The listing builds one solid part. Answer for the finished solid, in the listing's coordinates (mm). Face numbers are marked on the shaded views. A direction names the side the tool comes from. Round coordinates to 2 decimals unless told otherwise and drop trailing zeros. Order: outer loops, then holes, each group sorted by start corner. A loop starts at its lowest first (then second) coordinate and runs counter-clockwise, first axis right, second up. Notation, with made-up numbers: (39.5, -7) - (66.5, -7) arc R25 ccw to (66.5, 13) - close; hole circle Ø2 at (39.5, -17). An arc over 180 degrees is marked (long way). One line per item, written item: value. Start each with the question number.
1. A tool of negligible diameter and unlimited length cuts with its end or side. For the marked faces 1, 2 and 3, from which of +Z, -Z, +X, -X, +Y, -Y can it reach the whole face along a straight path? Write none if from no direction.
2. Straight lines are drawn through the part: line 1 (X direction, y = 1, z = 1.75); line 2 (Y direction, x = 21, z = 2.5); line 3 (Z direction, x = 51.5, y = 2). For each, find the intervals that lie inside material, in ascending order.
3. Section C-C, the plane x = -70 is taken. Give the vertices of the cut face in (y, z), then the cut area to 3 significant figures.
4. Flat-ended cylindrical pins translate along their axes: P1, Ø9, axis at x = 56.77, y = -1.58, coming from the -Z side; P2, Ø0.8, axis at y = 7, z = 3, coming from the +X side; P3, Ø1.5, axis at x = -102.5, z = 4.5, coming from the +Y side; P4, Ø1.2, axis at y = 7, z = 6, coming from the -X side. Find the tip coordinate at first contact, or state that the pin passes through.
5. Section B-B, the plane x = 42 is taken. Give the vertices of the cut face in (y, z).
6. Section A-A, the plane z = 3.25 is taken. Give the vertices of the cut face in (x, y) (3 decimals).
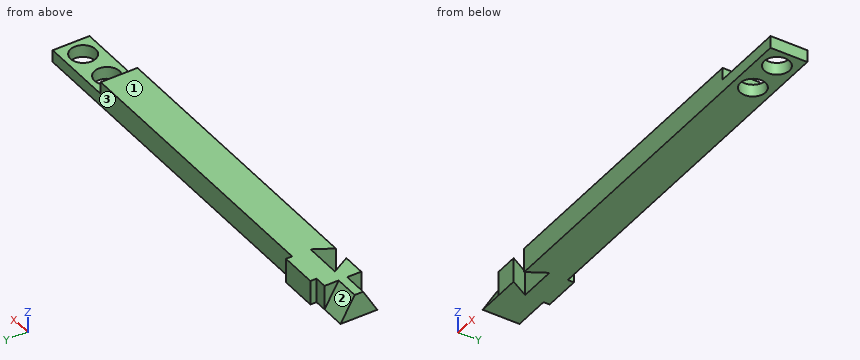
from build123d import *

# Parameters (mm, degrees)
SKETCH_W        = 170
SKETCH_H        = 15
PAD_DEPTH       = 10
SKETCH001_W     = 35
SKETCH001_H     = 25
POCKET_DEPTH    = 5
PAD002_DEPTH    = 10
POCKET001_DEPTH = 10
SKETCH002_R     = 5.125
POCKET002_DEPTH = 5
SKETCH005_W     = 15.25
SKETCH005_H     = 10
PAD003_DEPTH    = 2.5


with BuildPart() as part:
    # Sketch → Pad (new body)
    with BuildSketch(Plane.XY):
        with Locations((-20.728933, -1.58076)):
            Rectangle(SKETCH_W, SKETCH_H)
    extrude(amount=PAD_DEPTH)

    # Sketch001 (on Face6 of Pad) → Pocket (cut)
    with BuildSketch(Plane.XY.offset(10)):
        with Locations((51.771067, -1.58076)):
            Rectangle(SKETCH001_W, SKETCH001_H)
    extrude(amount=-POCKET_DEPTH, mode=Mode.SUBTRACT)

    # Sketch003 → Pad002 (join)
    with BuildSketch(Plane(origin=(-105.728933, 0, 0), x_dir=(0, -1, 0), z_dir=(-1, 0, 0))):
        Polygon((-5.91924, 0), (-0.145737, 10), (3.307257, 10), (9.08076, 0), align=None)
    extrude(amount=PAD002_DEPTH)

    # Sketch004 (on Face3 of Pad002) → Pocket001 (cut)
    with BuildSketch(Plane.XY.offset(10)):
        Polygon((-93.103933, -14.787648), (-100.728933, -1.58076), (-85.478933, -1.58076), align=None)
    extrude(amount=-POCKET001_DEPTH, mode=Mode.SUBTRACT)

    # Sketch002 (on Face7 of Pocket) → Pocket002 (cut)
    with BuildSketch(Plane.XY.offset(5)):
        with Locations((56.771067, -1.58076)):
            Circle(SKETCH002_R)
        with Locations((41.771067, -1.58076)):
            Circle(SKETCH002_R)
    extrude(amount=-POCKET002_DEPTH, mode=Mode.SUBTRACT)

    # Sketch005 (on Face9 of Pocket002) → Pad003 (join)
    with BuildSketch(Plane(origin=(0, 5.91924, 0), x_dir=(-1, 0, 0), z_dir=(0, 1, 0))):
        with Locations((93.103933, 5)):
            Rectangle(SKETCH005_W, SKETCH005_H)
    extrude(amount=PAD003_DEPTH)


solid = part.part
Answer list:
1. face 1: +Z, +X, -X, +Y, -Y
1. face 2: +Z, -X, +Y
1. face 3: +Z, -Z, +X, +Y
2. line 1: x = -115.73 to 37.34, 46.2 to 52.34, 61.2 to 64.27
2. line 2: y = -9.08 to 5.92
2. line 3: z = 0 to 5
3. outline: (-9.08, 0) - (5.92, 0) - (5.92, 10) - (-9.08, 10) - close
3. area: 150 mm²
4. P1: passes through
4. P2: stops at x = -85.48
4. P3: stops at y = 5.92
4. P4: stops at x = -100.73
5. outline: (-9.08, 0) - (-6.7, 0) - (-6.7, 5) - (-9.08, 5) - close; (3.54, 0) - (5.92, 0) - (5.92, 5) - (3.54, 5) - close
6. outline: (-115.729, -7.204) - (-105.729, -7.204) - (-105.729, -9.081) - (-96.399, -9.081) - (-100.729, -1.581) - (-85.479, -1.581) - (-89.809, -9.081) - (64.271, -9.081) - (64.271, 5.919) - (-85.479, 5.919) - (-85.479, 8.419) - (-100.729, 8.419) - (-100.729, 5.919) - (-105.729, 5.919) - (-105.729, 4.043) - (-115.729, 4.043) - close; hole circle Ø10.25 at (41.771, -1.581); hole circle Ø10.25 at (56.771, -1.581)
